Build history of the part. All positions in model axes, mm. A direction names the side the tool comes from. Round coordinates to 2 decimals unless told otherwise and drop trailing zeros. Write each loop counter-clockwise with the first axis right and the second up, starting at its lowest first coordinate (ties: lowest second). Pieces come first, ordered by that corner, then holes. Notation, with made-up numbers: M -16,85.5 L 30,85.5 A37 ccw 30,122.5 Z; hole C -26.5,80.25 d2. An arc over 180 degrees is marked long. Write item = value, one per line. Start each with the question number.
Q1. Drop flat-ended pins along their axis: P1, Ø8, axis at x = -15, y = 10.5, coming from the -Z side; P2, Ø7.5, axis at y = 0, z = 20, coming from the +X side; P3, Ø8, axis at x = 17, y = 17, coming from the +Z side; P4, Ø3, axis at y = -12.5, z = 25, coming from the +X side. Give the stop position or say it passes through.
Q2. Probe L1, parallel to X at y = -17, z = 30; L2, parallel to Y at x = -20, z = 5.5. List the from-to ranges inside material, lowest first.
Q3. Band-saw the part on A-A on z = 95. Write the cut outline in (x, y).
Q4. Pull direction Y, two halves, no side cores. Call faces 4 (the flat face through (0, -22.5, 57)), 5 (the flat face through (20, 0, 95)), 6 (the flat face through (27, 0, 58)): released by +Y, released by -Y, zero draft, split by the parting line, or undercut.
Q5. Tool access for faces 1 (the flat face through (17, -20, 7)), 2 (the cylindrical face through (-1.756, -7.907, 111.451)), 3 (the flat face through (20, 0, 20)): list every direction of +Z, -Z, +X, -X, +Y, -Y with a clear straight run to the whole face (end or side of a thin tool).
Q6. Band-saw the part on C-C on x = 0. Write the cut outline in (y, z).
Q7. Band-saw the part on D-D on z = 58.5. Write the cut outline in (x, y), plus the area to 3 significant figures.
Q8. Band-saw the part on B-B on y = 10.5. Write the cut outline in (x, z), plus the area to 3 significant figures.
```python
from build123d import *

# Parameters (mm, degrees)
SKETCH1_W                                      = 45
SKETCH1_H                                      = 45
SKETCH1_R                                      = 2.75
SKETCH1_R_2                                    = 16
SMC_45_MM_SQUARE_BODY_AND_FOUR_5_5_MM_TH_DEPTH = 115
SKETCH2_R                                      = 16
HEAD_END_CLEARANCE_ENVELOPE_DEPTH              = 7
ROD_START                                      = 108
SKETCH3_R                                      = 16
SKETCH3_R_2                                    = 8.1
ROD_COVER_AND_16_MM_ROD_CLEARANCE_DEPTH        = 7
SKETCH4_R                                      = 4.5
REAR_BOLT_HEAD_COUNTERBORES_DEPTH              = 7
FRONT_START                                    = 108
SKETCH5_R                                      = 4.5
FRONT_MOUNTING_COUNTERBORES_DEPTH              = 7
CATALOG_START                                  = 22.4
SKETCH6_W                                      = 115
SKETCH6_H                                      = 14
CATALOG_14_MM_WIDE_PORT_BOSS_PROJECTION_DEPTH  = 4.6
TOP_START                                      = 27
SKETCH7_R                                      = 4.55
TOP_RC_1_8_PORTS_20_MM_FROM_EACH_END_DEPTH     = 7


with BuildPart() as part:
    # Sketch1 → SMC 45 mm square body and four 5.5 mm through holes (new body)
    with BuildSketch(Plane.XY):
        Rectangle(SKETCH1_W, SKETCH1_H)
        with Locations((-17, -17)):
            Circle(SKETCH1_R, mode=Mode.SUBTRACT)
        with Locations((-17, 17)):
            Circle(SKETCH1_R, mode=Mode.SUBTRACT)
        with Locations((17, -17)):
            Circle(SKETCH1_R, mode=Mode.SUBTRACT)
        with Locations((17, 17)):
            Circle(SKETCH1_R, mode=Mode.SUBTRACT)
        Circle(SKETCH1_R_2, mode=Mode.SUBTRACT)
    extrude(amount=SMC_45_MM_SQUARE_BODY_AND_FOUR_5_5_MM_TH_DEPTH)

    # Sketch2 → Head end clearance envelope (add)
    with BuildSketch(Plane.XY):
        Circle(SKETCH2_R)
    extrude(amount=HEAD_END_CLEARANCE_ENVELOPE_DEPTH)

    # Sketch3 → Rod cover and 16 mm rod clearance (add)
    with BuildSketch(Plane.XY.offset(ROD_START)):
        Circle(SKETCH3_R)
        Circle(SKETCH3_R_2, mode=Mode.SUBTRACT)
    extrude(amount=ROD_COVER_AND_16_MM_ROD_CLEARANCE_DEPTH)

    # Sketch4 → Rear bolt head counterbores (cut)
    with BuildSketch(Plane.XY):
        with Locations((-17, -17)):
            Circle(SKETCH4_R)
        with Locations((-17, 17)):
            Circle(SKETCH4_R)
        with Locations((17, -17)):
            Circle(SKETCH4_R)
        with Locations((17, 17)):
            Circle(SKETCH4_R)
    extrude(amount=REAR_BOLT_HEAD_COUNTERBORES_DEPTH, mode=Mode.SUBTRACT)

    # Sketch5 → Front mounting counterbores (cut)
    with BuildSketch(Plane.XY.offset(FRONT_START)):
        with Locations((-17, -17)):
            Circle(SKETCH5_R)
        with Locations((-17, 17)):
            Circle(SKETCH5_R)
        with Locations((17, -17)):
            Circle(SKETCH5_R)
        with Locations((17, 17)):
            Circle(SKETCH5_R)
    extrude(amount=FRONT_MOUNTING_COUNTERBORES_DEPTH, mode=Mode.SUBTRACT)

    # Sketch6 → Catalog 14 mm wide port boss projection (add)
    with BuildSketch(Plane(origin=(0, 0, 0), x_dir=(0, 0, -1), z_dir=(1, 0, 0)).offset(CATALOG_START)):
        with Locations((-57.5, 0)):
            Rectangle(SKETCH6_W, SKETCH6_H)
    extrude(amount=CATALOG_14_MM_WIDE_PORT_BOSS_PROJECTION_DEPTH)

    # Sketch7 → Top Rc 1/8 ports, 20 mm from each end (cut)
    with BuildSketch(Plane(origin=(0, 0, 0), x_dir=(0, 0, -1), z_dir=(1, 0, 0)).offset(TOP_START)):
        with Locations((-20, 0)):
            Circle(SKETCH7_R)
        with Locations((-95, 0)):
            Circle(SKETCH7_R)
    extrude(amount=-TOP_RC_1_8_PORTS_20_MM_FROM_EACH_END_DEPTH, mode=Mode.SUBTRACT)


solid = part.part
```
Conclusion:
q1.P1 = 0
q1.P2 = 20
q1.P3 = 108
q1.P4 = 22.5
q2.L1 = -22.5 to -19.75, -14.25 to 14.25, 19.75 to 22.5
q2.L2 = -22.5 to -20.35, -13.65 to 13.65, 20.35 to 22.5
q3.outline = M -22.5,-22.5 L 22.5,-22.5 L 22.5,-7 L 27,-7 L 27,-4.55 L 20,-4.55 L 20,4.55 L 27,4.55 L 27,7 L 22.5,7 L 22.5,22.5 L -22.5,22.5 Z; hole C -17,-17 d5.5; hole C -17,17 d5.5; hole C 0,0 d32; hole C 17,-17 d5.5; hole C 17,17 d5.5
q4.face_4 = released by -Y
q4.face_5 = undercut
q4.face_6 = zero draft
q5.face_1 = -Z
q5.face_2 = +Z
q5.face_3 = +X
q6.outline = M -22.5,0 L 22.5,0 L 22.5,115 L 8.1,115 L 8.1,108 L 16,108 L 16,7 L -16,7 L -16,108 L -8.1,108 L -8.1,115 L -22.5,115 Z
q7.outline = M -22.5,-22.5 L 22.5,-22.5 L 22.5,-7 L 27,-7 L 27,7 L 22.5,7 L 22.5,22.5 L -22.5,22.5 Z; hole C -17,-17 d5.5; hole C -17,17 d5.5; hole C 0,0 d32; hole C 17,-17 d5.5; hole C 17,17 d5.5
q7.area = 1,190 mm^2
q8.outline = M -22.5,0 L 22.5,0 L 22.5,115 L -22.5,115 Z; hole M -12.07,7 L 12.07,7 L 12.07,108 L -12.07,108 Z
q8.area = 2,740 mm^2
